Autodesk Inventor part; units mm, degrees
ref_plane "YZ Plane" through (0, 0, 0) normal (1, 0, 0) x (0, 1, 0)
ref_plane "XZ Plane" through (0, 0, 0) normal (0, 1, 0) x (-1, 0, 0)
ref_plane "XY Plane" through (0, 0, 0) normal (0, 0, 1) x (1, 0, 0)
sketch "Sketch1" plane through (0, 0, 0) normal (0, 1, 0) x (-1, 0, 0)
  line L0 (0, 0) -> (0, -2.5)
  line L1 (0, 0) -> (-8.2, 0)
  line L2 (-8.2, 0) -> (-8.2, -2.3)
  line L3 (-8.2, -2.3) -> (-6.7, -2.3)
  line L4 (0, -2.5) -> (-1.5, -2.5)
  line L5 (-1.5, -2.5) -> (-1.5, -5)
  line L6 (-6.7, -2.3) -> (-6.7, -4.8)
  line L7 (-6.7, -4.8) -> (-13.6, -4.8)
  line L8 (-13.6, -4.8) -> (-13.6, -20.8)
  line L9 (-1.5, -5) -> (0, -5)
  line L10 (-13.6, -20.8) -> (0, -20.8)
  line L11 (0, -20.8) -> (0, -5)
  dimension "d0" = 2.5
  dimension "d1" = 8.2
  dimension "d2" = 2.3
  dimension "d3" = 1.5
  dimension "d4" = 1.5
  dimension "d5" = 2.5
  dimension "d6" = 2.5
  dimension "d7" = 6.9
  dimension "d8" = 16
extrude "Extrusion1" add sketch "Sketch1" along normal blind 142
sketch "Sketch2" plane through (0, 0, -20.8) normal (-1, 0, 0) x (0, 0, 1)
  line L0 (0, 142) -> (15.8, 142)
  line L1 (0, 0) -> (15.8, 0)
  point P0 (20.8, 0)
  point P1 (8, 131)
  point P2 (8, 11)
  point P3 (7.9, 51)
  point P4 (7.9, 91)
  dimension "d11" = 11
  dimension "d12" = 11
  dimension "d13" = 40
  dimension "d14" = 40
hole "Hole1" at (0, 131, -12.8) at (0, 11, -12.8) at (0, 51, -12.9) at (0, 91, -12.9) direction (1, 0, 0) diameter 6.604 end through all counterbore diameter 10.9982 counterbore depth 5.9944
properties part number "aactuatorHolder" material "ABS Plastic"
Verification items for the finished model (mm, model axes). A direction names the side the tool comes from. Coordinates: 2 decimals unless noted, no trailing zeros. Loops run counter-clockwise (first coordinate to the right, second up) from the corner with the lowest first, then second, coordinate; pieces in that order, holes last. Notation, with made-up numbers: (24, -1.75) -> (69, -1.75) arc R34 ccw to (69, 37.25) -> close; hole circle Ø2 at (42.25, 2.25). An arc over 180 degrees is marked (long way). Put each result on its own line as item: value.
1. Tool access check on faces 5 (the face through (10, 70, -4.8)), 6 (the face through (0, 70, -1)), 7 (the face through (8.2, 70, -1)), 8 (the face through (1.5, 70, -4)), 9 (the face through (3.04, 96.37, -14.09)). Record the directions out of +Z, -Z, +X, -X, +Y, -Y that give a thin tool (end or side, any length) a straight path to the whole face; none if there is none.
Result set:
face 5: +X, +Y, -Y
face 6: +Z, -Z, -X, +Y, -Y
face 7: +Z, +X, +Y, -Y
face 8: -X, +Y, -Y
face 9: -X
2. Section check C-C, the plane y = 102.5. Record the boundary of the cut face in (x, z), then the cut area to 3 significant figures.
Result set:
outline: (0, -20.8) -> (13.6, -20.8) -> (13.6, -4.8) -> (6.7, -4.8) -> (6.7, -2.3) -> (8.2, -2.3) -> (8.2, 0) -> (0, 0) -> (0, -2.5) -> (1.5, -2.5) -> (1.5, -5) -> (0, -5) -> close
area: 249 mm^2
3. Section check A-A, the plane y = 131. Record the boundary of the cut face in (x, z), then the cut area to 3 significant figures.
Result set:
outline: (0, -20.8) -> (13.6, -20.8) -> (13.6, -16.1) -> (5.99, -16.1) -> (5.99, -18.3) -> (0, -18.3) -> close; (0, -7.3) -> (5.99, -7.3) -> (5.99, -9.5) -> (13.6, -9.5) -> (13.6, -4.8) -> (6.7, -4.8) -> (6.7, -2.3) -> (8.2, -2.3) -> (8.2, 0) -> (0, 0) -> (0, -2.5) -> (1.5, -2.5) -> (1.5, -5) -> (0, -5) -> close
area: 133 mm^2
4. Gauge pin test, flat ends, axial feed: P1, Ø2, axis at y = 23, z = -3.5, coming from the +X side; P2, Ø5.5, axis at y = 93, z = -14.5, coming from the -X side; P3, Ø2, axis at x = 11.5, y = 59.5, coming from the +Z side. Record the tip position at first contact, or that the pin passes through.
Result set:
P1: stops at x = 6.7
P2: stops at x = 5.99
P3: stops at z = -4.8
5. Section check B-B, the plane x = 3.5. Record the boundary of the cut face in (y, z), then the cut area to 3 significant figures.
Result set:
outline: (0, -20.8) -> (142, -20.8) -> (142, 0) -> (0, 0) -> close; hole circle Ø11 at (11, -12.8); hole circle Ø11 at (51, -12.9); hole circle Ø11 at (91, -12.9); hole circle Ø11 at (131, -12.8)
area: 2,570 mm^2
6. Mould release check, pull along Y, two halves, no side actions. Record for faces 1 (the face through (9.85, 88.22, -11.12)), 2 (the face through (0, 70, -13)), 3 (the face through (3.04, 16.37, -13.99)), 4 (the face through (7, 142, -10)): pulls with the +Y half, pulls with the -Y half, needs draft (parallel to the pull), parting line crosses it, or undercut.
Result set:
face 1: undercut
face 2: needs draft
face 3: undercut
face 4: pulls with the +Y half
7. Section check D-D, the plane x = 11.5. Record the boundary of the cut face in (y, z), then the cut area to 3 significant figures.
Result set:
outline: (0, -20.8) -> (142, -20.8) -> (142, -4.8) -> (0, -4.8) -> close; hole circle Ø6.6 at (11, -12.8); hole circle Ø6.6 at (51, -12.9); hole circle Ø6.6 at (91, -12.9); hole circle Ø6.6 at (131, -12.8)
area: 2,130 mm^2
8. Thickness scan on line 1 (Z direction, x = 8, y = 51); line 2 (Z direction, x = 1.45, y = 91); line 3 (Y direction, x = 9, z = -12.9). Record the ranges inside material, lowest first.
Result set:
line 1: z = -20.8 to -16.2, -9.6 to -4.8, -2.3 to 0
line 2: z = -20.8 to -18.4, -7.4 to -5, -2.5 to 0
line 3: y = 0 to 7.7, 14.3 to 47.7, 54.3 to 87.7, 94.3 to 127.7, 134.3 to 142
